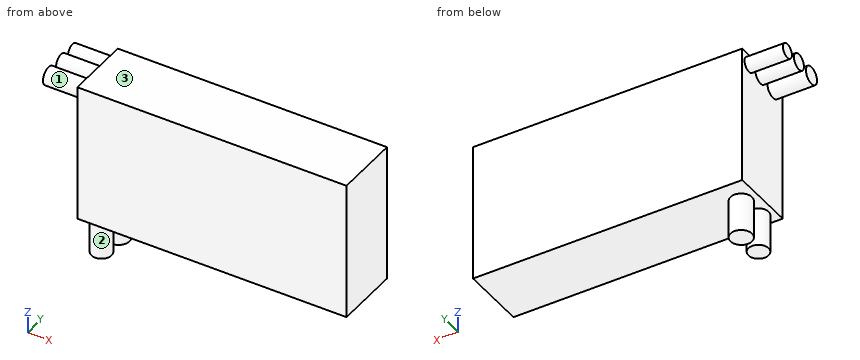
from build123d import *

# Parameters (mm, degrees)
SKETCH3_W           = 70
SKETCH3_H           = 36
BOSS_EXTRUDE2_DEPTH = 17
SKETCH4_R           = 1.880557467
SKETCH4_R_2         = 2.098035393
SKETCH4_R_3         = 2.319039591
BOSS_EXTRUDE3_DEPTH = 10
SKETCH5_R           = 2.614216035
SKETCH5_R_2         = 2.802234852
BOSS_EXTRUDE4_DEPTH = 10


with BuildPart() as part:
    # Sketch3 → Boss-Extrude2 (new body)
    with BuildSketch(Plane(origin=(0, 0, 0), x_dir=(1, 0, 0), z_dir=(0, 1, 0))):
        Rectangle(SKETCH3_W, SKETCH3_H)
    extrude(amount=BOSS_EXTRUDE2_DEPTH)

    # Sketch4 → Boss-Extrude3 (add)
    with BuildSketch(Plane.ZY.offset(35)):
        with Locations(Location((15.274859304, 14.166430081, 0), (0, 0, 180))):
            Circle(SKETCH4_R)
        with Locations(Location((15.274859304, 9.332242636, 0), (0, 0, 180))):
            Circle(SKETCH4_R_2)
        with Locations(Location((14.82177003, 4.074871994, 0), (0, 0, 180))):
            Circle(SKETCH4_R_3)
    extrude(amount=BOSS_EXTRUDE3_DEPTH)

    # Sketch5 → Boss-Extrude4 (add)
    with BuildSketch(Plane(origin=(0, 0, -18), x_dir=(-1, 0, 0), z_dir=(0, 0, -1))):
        with Locations(Location((31.106031622, 3.885850759, 0), (0, 0, 180))):
            Circle(SKETCH5_R)
        with Locations(Location((30.683181336, 10.433921975, 0), (0, 0, 180))):
            Circle(SKETCH5_R_2)
    extrude(amount=BOSS_EXTRUDE4_DEPTH)


solid = part.part
The listing builds one solid part. Answer for the finished solid, in the listing's coordinates (mm). Face numbers are marked on the shaded views. A direction names the side the tool comes from. Coordinates: 2 decimals unless noted, no trailing zeros. Write each loop counter-clockwise with the first axis right and the second up, starting at its lowest first coordinate (ties: lowest second). Pieces come first, ordered by that corner, then holes. Notation, with made-up numbers: (-17, -10.5) - (-3, -10.5) arc R21 ccw to (-3, -1.5) - close; hole circle Ø1 at (89.5, 56). An arc over 180 degrees is marked (long way). Put each result on its own line as item: value.
1. The part is cut by section C-C on y = 2.75. Give the vertices of the cut face in (x, z), plus the area to 3 significant figures.
Answer sheet:
outline: (-45, 12.92) - (-35, 12.92) - (-35, -18) - (-33.46, -18) - (-33.46, -28) - (-28.75, -28) - (-28.75, -18) - (35, -18) - (35, 18) - (-35, 18) - (-35, 16.73) - (-45, 16.73) - close
area: 2,610 mm^2
2. The part is cut by section A-A on x = -12. Give the vertices of the cut face in (y, z), plus the area to 3 significant figures.
Answer sheet:
outline: (0, -18) - (17, -18) - (17, 18) - (0, 18) - close
area: 612 mm^2
3. Find the intervals of material crossed by line 1 along Z through (x, y) = (-11.5, 15.5); line 2 along X through (y, z) = (8, 9.5); line 3 along X through (y, z) = (5.75, -24), in increasing order. Write a range as from..to.
Answer sheet:
line 1: z = -18..18
line 2: x = -35..35
line 3: x = -32.94..-29.27
4. The part is cut by section B-B on z = -1. Give the vertices of the cut face in (x, y), plus the area to 3 significant figures.
Answer sheet:
outline: (-35, 0) - (35, 0) - (35, 17) - (-35, 17) - close
area: 1,190 mm^2
5. A tool of negligible diameter and unlimited length cuts with its end or side. For the marked faces 1, 2 and 3, from which of +Z, -Z, +X, -X, +Y, -Y can it reach the whole face along a straight path? Write none if from no direction.
Answer sheet:
face 1: -X
face 2: -Z
face 3: +Z, +X, -X, +Y, -Y
6. Flat-ended cylindrical pins translate along their axes: pin 1 Ø1.5 at (x, z) = (-31.5, -23) entering from -Y; pin 2 Ø4 at (y, z) = (3.5, -21.5) entering from -X; pin 3 Ø10 at (x, y) = (-4, 7) entering from -Z; pin 4 Ø8 at (x, z) = (1.5, 2.5) entering from -Y. Find the tip coordinate at first contact, or state that the pin passes through.
Answer sheet:
pin 1: stops at y = 1.27
pin 2: stops at x = -33.72
pin 3: stops at z = -18
pin 4: stops at y = 0
7. The part is cut by section D-D on z = -20.5. Give the vertices of the cut face in (x, y), plus the area to 3 significant figures.
Answer sheet:
outline: circle Ø5.23 at (-31.11, 3.89); circle Ø5.6 at (-30.68, 10.43)
area: 46.1 mm^2
